Autodesk Inventor part; units mm, degrees
ref_plane "YZ Plane" through (0, 0, 0) normal (1, 0, 0) x (0, 1, 0)
ref_plane "XZ Plane" through (0, 0, 0) normal (0, 1, 0) x (-1, 0, 0)
ref_plane "XY Plane" through (0, 0, 0) normal (0, 0, 1) x (1, 0, 0)
sketch "スケッチ1" plane through (0, -85.3303, 0) normal (0, 0, 1) x (1, 0, 0)
  circle A0 centre (0, 85.3303) radius 5 construction
  line L0 (10.253, 75.0773) -> (-10.253, 75.0773) construction
  line L1 (-10.253, 75.0773) -> (-10.253, 95.5834) construction
  line L2 (-10.253, 95.5834) -> (10.253, 95.5834) construction
  line L3 (10.253, 95.5834) -> (10.253, 75.0773) construction
  line L4 (10.253, 75.0773) -> (-10.253, 95.5834) construction
  line L5 (-10.253, 75.0773) -> (10.253, 95.5834) construction
  circle A1 centre (-10.253, 95.5834) radius 1.65
  circle A2 centre (-10.253, 75.0773) radius 1.65
  circle A3 centre (10.253, 75.0773) radius 1.65
  circle A4 centre (10.253, 95.5834) radius 1.65
  circle A5 centre (0, 85.3303) radius 9.5
  line L6 (-15.5, 52.3303) -> (-12.5, 52.3303)
  line L7 (-12.5, 46.3303) -> (-15.5, 46.3303)
  line L8 (-15.5, 46.3303) -> (-15.5, 52.3303)
  line L9 (-15.5, 38.3303) -> (-12.5, 38.3303)
  line L10 (-12.5, 32.3303) -> (-15.5, 32.3303)
  line L11 (-15.5, 32.3303) -> (-15.5, 38.3303)
  line L12 (-15.5, 24.3303) -> (-12.5, 24.3303)
  line L13 (-12.5, 18.3303) -> (-15.5, 18.3303)
  line L14 (-15.5, 18.3303) -> (-15.5, 24.3303)
  arc A6 (-12.5, 24.3303) -> (-12.5, 26.3303) centre (-12.5, 25.3303) ccw
  arc A7 (-12.5, 30.3303) -> (-12.5, 32.3303) centre (-12.5, 31.3303) ccw
  arc A8 (-12.5, 38.3303) -> (-12.5, 40.3303) centre (-12.5, 39.3303) ccw
  arc A9 (-12.5, 44.3303) -> (-12.5, 46.3303) centre (-12.5, 45.3303) ccw
  line L15 (-12.5, 44.3303) -> (-12.5, 40.3303)
  line L16 (-12.5, 30.3303) -> (-12.5, 26.3303)
  arc A10 (-12.5, 52.3303) -> (-11.5677, 53.692) centre (-12.5, 53.3303) ccw
  line L17 (-18.5, 100.5834) -> (0, 100.5834)
  line L18 (0, 100.5834) -> (0, 94.8303)
  line L19 (5, 15.3303) -> (-5, 15.3303)
  line L20 (-5, 15.3303) -> (-5, 18.6303)
  line L21 (5, 18.6303) -> (-5, 18.6303)
  line L22 (5, 15.3303) -> (5, 18.6303)
  arc A11 (0, 20.3336) -> (-6.25, 19.3319) centre (0, 0.3336) ccw
  line L23 (0, 20.3336) -> (0, 75.8303)
  arc A12 (-12.5, 18.3303) -> (-6.25, 19.3319) centre (-12.5, 38.3303) ccw
  line L24 (-18.5, 94.5834) -> (-15.5, 94.5834)
  line L25 (-15.5, 92.5834) -> (-15.5, 82.5834)
  line L26 (-15.5, 80.5834) -> (-18.5, 80.5834)
  line L27 (-18.5, 82.5834) -> (-18.5, 92.5834)
  arc A13 (-18.5, 94.5834) -> (-18.5, 92.5834) centre (-18.5, 93.5834) ccw
  arc A14 (-18.5, 82.5834) -> (-18.5, 80.5834) centre (-18.5, 81.5834) ccw
  arc A15 (-15.5, 80.5834) -> (-15.5, 82.5834) centre (-15.5, 81.5834) ccw
  arc A16 (-15.5, 92.5834) -> (-15.5, 94.5834) centre (-15.5, 93.5834) ccw
  circle A17 centre (-21.5, 87.5834) radius 1.25
  arc A18 (-24.4541, 87.0604) -> (-24.2968, 86.4981) centre (-21.5, 87.5834) ccw
  line L28 (-25.3928, 92.3631) -> (-24.4541, 87.0604)
  line L29 (-24.2968, 86.4981) -> (-11.5677, 53.692)
  arc A19 (-18.5, 100.5834) -> (-25.3928, 92.3631) centre (-18.5, 93.5834) ccw
  line L30 (0, 58.3303) -> (-1.5, 58.3303)
  line L31 (-1.5, 60.3303) -> (-1.5, 70.3303)
  line L32 (-1.5, 72.3303) -> (0, 72.3303)
  arc A20 (-1.5, 72.3303) -> (-1.5, 70.3303) centre (-1.5, 71.3303) ccw
  arc A21 (-1.5, 60.3303) -> (-1.5, 58.3303) centre (-1.5, 59.3303) ccw
  circle A22 centre (-4.5, 65.3303) radius 1.25
  point P0 (0, 85.3303)
  point P1 (-15.5, 87.5834)
  point P2 (-1.5, 65.3303)
  dimension "d0" = 29
  dimension "d1" = 3.3
  dimension "d4" = 360
  dimension "d6" = 19
  dimension "d7" = 15.5
  dimension "d8" = 33
  dimension "d9" = 8
  dimension "d10" = 6
  dimension "d11" = 8
  dimension "d12" = 3
  dimension "d13" = 1
  dimension "d16" = 6
  dimension "d17" = 20
  dimension "d19" = 20
  dimension "d24" = 15.5
  dimension "d26" = 3
  dimension "d27" = 2
  dimension "d28" = 14
  dimension "d31" = 18.5
  dimension "d32" = 5
  dimension "d33" = 2.5
  dimension "d34" = 3
  dimension "d35" = 6
  dimension "d36" = 6
  dimension "d37" = 14
  dimension "d38" = 1.5
  dimension "d39" = 2.5
  dimension "d40" = 3
  dimension "d41" = 20
extrude "押し出し2" add sketch "スケッチ1" along normal blind 3 contours A5 L23 L32 A20 L31 A21 L30 A11 A12 L13 L14 L12 A6 L16 A7 L10 L11 L9 A8 L15 A9 L7 L8 L6 A10 L29 A18 L28 A19 L17 L18
mirror "ミラー2" about plane through (0, -13, 0) normal (1, 0, 0) of "押し出し2"
equation "\"d11\" = d9"
equation "\"d37\" = d28"
properties part number "スライダベアリングハウジング"
Design review of the part built by this model. Coordinates are the model's own, in mm. A direction names the side the tool comes from. Give positions to 0.01 mm unless a question says otherwise; leave off trailing zeros. Order: outer loops, then holes, each group sorted by start corner. A loop starts at its lowest first (then second) coordinate and runs counter-clockwise, first axis right, second up.
1. Add section A-A, the plane y = -40. State the section outline as (x, z) points, then the cut area to 3 significant figures.
Solution:
outline: (-11.5, 0) - (11.5, 0) - (11.5, 3) - (-11.5, 3) - close
area: 69.0 mm2
2. Add section C-C, the plane y = -52. State the section outline as (x, z) points, then the cut area to 3 significant figures.
Solution:
outline: (-15.5, 0) - (15.5, 0) - (15.5, 3) - (-15.5, 3) - close
area: 93.0 mm2
3. Tool access review of faces 1 (the flat face through (-15.5, 2, 1)), 2 (the flat face through (14, -47, 1)), 3 (the flat face through (-14, -33, 1)): name each direction out of +Z, -Z, +X, -X, +Y, -Y from which nothing blocks a thin tool from reaching the whole face with its end or side.
Solution:
face 1: +Z, -Z
face 2: +Z, -Z, +X
face 3: +Z, -Z, -X
4. Mouldability with a two-part tool opening along Y and no side actions: class faces 4 (the flat face through (-15.5, -36, 1)), 5 (the cylindrical face through (4.77, -21.22, 1.48)), 6 (the cylindrical face through (9.379, -66.755, 1.479)) as +Y half, -Y half, draft (parallel to the pull), parting line (faces both ways), or undercut.
Solution:
face 4: draft
face 5: undercut
face 6: -Y half
5. To check wall thickness, follow L1, parallel to X at y = 0, z = 2.2; L2, parallel to Y at x = 10, z = 2.75; L3, parallel to Y at x = 11, z = 2.3. State the ranges of each line that lie inside material, in increasing order.
Solution:
L1: x = -23.84 to -18.5, -15.5 to -9.5, 9.5 to 15.5, 18.5 to 23.84
L2: y = -66.84 to -11.88, -8.62 to 8.62, 11.88 to 15.25
L3: y = -66.94 to -11.72, -8.78 to 8.78, 11.72 to 15.25
6. Add section B-B, the plane z = 0.9. State how many separate pieces and enclosed holes the cut face has, then the cut area to 3 significant figures.
Solution:
separate pieces: 1
enclosed holes: 12
area: 2,340 mm2
7. For pin 1 Ø0.9 at (y, z) = (-34.5, 1.5) entering from -X; pin 2 Ø3 at (x, y) = (-10.25, 10.25) entering from +Z; pin 3 Ø1.5 at (y, z) = (3, 1) entering from -X; pin 4 Ø1.5 at (y, z) = (-42.5, 1.5) entering from -X, all flat-tipped, find the tip position at first contact; note any pin that passes through.
Solution:
pin 1: stops at x = -15.5
pin 2: passes through
pin 3: stops at x = -24.81
pin 4: stops at x = -12.5
